Check sheet for the modelled part. Datum: model origin and axes. Units: mm. Give positions to 0.01 mm unless a question says otherwise; leave off trailing zeros. Loops run counter-clockwise (first coordinate to the right, second up) from the corner with the lowest first, then second, coordinate; pieces in that order, holes last. Notation, with made-up numbers: M 45,25 L 87,25 A18 cw 87,54 Z; hole C 69.25,29 d4. An arc over 180 degrees is marked long. One line per question, with ' | ' between items. Start each with the question number.
from build123d import *

# Parameters (mm, degrees)
CROQUIS1_W              = 41.4
CROQUIS1_H              = 20.7
SALIENTE_EXTRUIR1_DEPTH = 26
CROQUIS3_R              = 5.25
SALIENTE_EXTRUIR2_DEPTH = 1
REDONDEO1_R             = 0.4
CROQUIS5_R              = 4.35
CORTAR_EXTRUIR1_DEPTH   = 0.1
REDONDEO2_R             = 1.2


with BuildPart() as part:
    # Croquis1 → Saliente-Extruir1 (new body)
    with BuildSketch(Plane(origin=(0, 0, 0), x_dir=(1, 0, 0), z_dir=(0, 1, 0))):
        Rectangle(CROQUIS1_W, CROQUIS1_H)
    extrude(amount=SALIENTE_EXTRUIR1_DEPTH)

    # Croquis3 → Saliente-Extruir2 (add)
    with BuildSketch(Plane.ZY.offset(20.7)):
        with Locations((0, 10)):
            Circle(CROQUIS3_R)
    extrude(amount=SALIENTE_EXTRUIR2_DEPTH)

    # Redondeo1
    redondeo1_edges = [part.edges().sort_by_distance(p)[0] for p in [
        (-20.7, 10, -5.25),
        (-21.7, 10, -5.25),
    ]]
    fillet(redondeo1_edges, radius=REDONDEO1_R)

    # Croquis5 → Cortar-Extruir1 (cut)
    with BuildSketch(Plane.ZY.offset(21.7)):
        with Locations((0, 10)):
            Circle(CROQUIS5_R)
    extrude(amount=-CORTAR_EXTRUIR1_DEPTH, mode=Mode.SUBTRACT)

    # Redondeo2
    redondeo2_edges = [part.edges().sort_by_distance(p)[0] for p in [
        (20.7, 13, 10.35),
        (-20.7, 13, 10.35),
        (-20.7, 13, -10.35),
        (20.7, 13, -10.35),
    ]]
    fillet(redondeo2_edges, radius=REDONDEO2_R)


solid = part.part
Q1. Cross-section at B-B (z = -6.5). Record the cut outline in (x, y), and give its area (3 significant figures).
Q2. Depth check by flat-ended pin: P1, Ø5, axis at x = 14.5, z = -8, coming from the -Y side; P2, Ø4.5, axis at y = 9.5, z = -1.5, coming from the -X side. Enter the tip coordinate at first touch or a pass-through.
Q3. Material ranges on probe 1 along X at (y, z) = (16, -1.25); probe 2 along Y at (x, z) = (-21.65, 0); probe 3 along X at (y, z) = (10.75, 1), recorded low to high. Write a range as from..to.
Q4. Cross-section at A-A (y = 3). Record the cut outline in (x, z).
Q5. Draft check along Z on faces 1 (the flat face through (0, 13, 10.35)), 2 (the flat face through (-21.6, 10, 0)), 3 (the flat face through (20.7, 13, 0)). Enter one of: released by +Z, released by -Z, zero draft, split by the parting line, or undercut.
Solved:
1) outline: M -20.7,0 L 20.7,0 L 20.7,26 L -20.7,26 Z | area: 1,080 mm²
2) P1: stops at y = 0 | P2: stops at x = -21.6
3) probe 1: x = -20.7..20.7 | probe 2: y = 4.96..5.65, 14.35..15.04 | probe 3: x = -21.6..20.7
4) outline: M -20.7,-9.15 A1.2 ccw -19.5,-10.35 L 19.5,-10.35 A1.2 ccw 20.7,-9.15 L 20.7,9.15 A1.2 ccw 19.5,10.35 L -19.5,10.35 A1.2 ccw -20.7,9.15 Z
5) face 1: released by +Z | face 2: undercut | face 3: zero draft
